Could you check a few things on this model? Use its own coordinates, in mm. Face numbers are marked on the shaded views. A direction names the side the tool comes from. Coordinates: 2 decimals unless noted, no trailing zeros. Order: outer loops, then holes, each group sorted by start corner. A loop starts at its lowest first (then second) coordinate and runs counter-clockwise, first axis right, second up. Notation, with made-up numbers: (-14, 35) - (23, 35) arc R22 ccw to (23, 44) - close; hole circle Ø9 at (-34.5, 37.5). An arc over 180 degrees is marked (long way). One line per item, written item: value.
from build123d import *

# Parameters (mm, degrees)
BOSS_EXTRUDE1_DEPTH = 67.056
SKETCH3_R           = 3.175
CUT_EXTRUDE1_DEPTH  = 16.875
SKETCH4_R           = 1.7500092
CUT_EXTRUDE2_DEPTH  = 16.875


with BuildPart() as part:
    # Sketch2 → Boss-Extrude1 (new body, symmetric)
    with BuildSketch(Plane.XY):
        with BuildLine():
            Line((-7.9375, 0), (7.9375, 0))
            Line((7.9375, 0), (7.9375, 15.875))
            Line((7.9375, 15.875), (7.14375, 15.875))
            ThreePointArc((7.14375, 15.875), (6.582483992, 15.642516008), (6.35, 15.08125))
            Line((6.35, 15.08125), (6.35, 2.38125))
            ThreePointArc((6.35, 2.38125), (6.117516008, 1.819983992), (5.55625, 1.5875))
            Line((5.55625, 1.5875), (-7.14375, 1.5875))
            ThreePointArc((-7.14375, 1.5875), (-7.705016008, 1.355016008), (-7.9375, 0.79375))
            Line((-7.9375, 0.79375), (-7.9375, 0))
        make_face()
    extrude(amount=BOSS_EXTRUDE1_DEPTH, both=True)

    # Sketch3 → Cut-Extrude1 (cut, through all)
    with BuildSketch(Plane(origin=(7.9375, 0, 0), x_dir=(0, 0, -1), z_dir=(1, 0, 0))):
        with Locations((-25.4, 7.9375)):
            Circle(SKETCH3_R)
        with Locations((25.4, 7.9375)):
            Circle(SKETCH3_R)
    extrude(amount=-CUT_EXTRUDE1_DEPTH, mode=Mode.SUBTRACT)

    # Sketch4 → Cut-Extrude2 (cut, through all)
    with BuildSketch(Plane.XZ):
        with Locations((0, -59.1185)):
            Circle(SKETCH4_R)
        with Locations((0, 59.1185)):
            Circle(SKETCH4_R)
    extrude(amount=-CUT_EXTRUDE2_DEPTH, mode=Mode.SUBTRACT)


solid = part.part
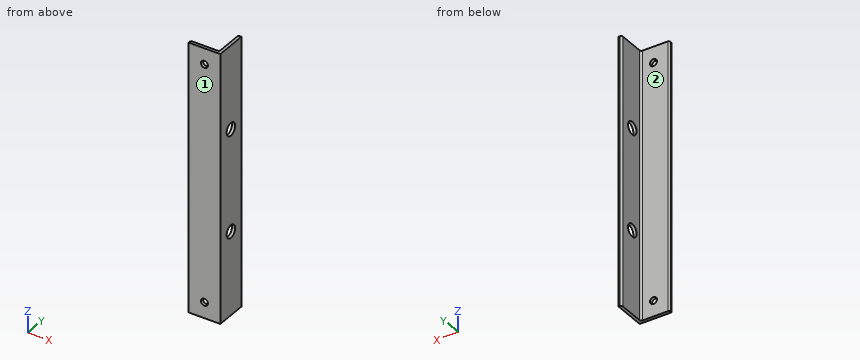
Item 1: If I drill on probe 1 along Z at (x, y) = (0, 0.85); probe 2 along Y at (x, z) = (7.2, 25.4) (1 decimal); probe 3 along X at (y, z) = (14.5, -21), over which ranges is the centre line in solid material (lowest first)?
Conclusion:
probe 1: -67.06 to -60.87, -57.37 to 57.37, 60.87 to 67.06
probe 2: 0 to 4.8, 11.1 to 15.9
probe 3: 6.35 to 7.94
Item 2: For the marked faces 1 and 2, which set-ups out of +Z, -Z, +X, -X, +Y, -Y let a thin tool reach every point of the face, with its end or its side?
Conclusion:
face 1: +Z, -Z, +X, -X, -Y
face 2: +Z, -Z, -X, +Y
Item 3: I want a section at D-D on y = 13.5. Please give me the cut outline in (x, z), then the cut area to 3 significant figures.
Conclusion:
outline: (6.35, -67.06) - (7.94, -67.06) - (7.94, 67.06) - (6.35, 67.06) - close
area: 213 mm²
Item 4: I'm going to push a flat-ended pin straight in: pin 1 Ø1.5 at (x, z) = (-5.5, 24) entering from +Y. Where does the tip first touch, or does it pass through?
Conclusion:
pin 1: y = 1.59
Item 5: I want a section at B-B on x = 0. Please give me the cut outline in (y, z), then the cut area to 3 significant figures.
Conclusion:
outline: (0, -67.06) - (1.59, -67.06) - (1.59, -60.87) - (0, -60.87) - close; (0, -57.37) - (1.59, -57.37) - (1.59, 57.37) - (0, 57.37) - close; (0, 60.87) - (1.59, 60.87) - (1.59, 67.06) - (0, 67.06) - close
area: 202 mm²
